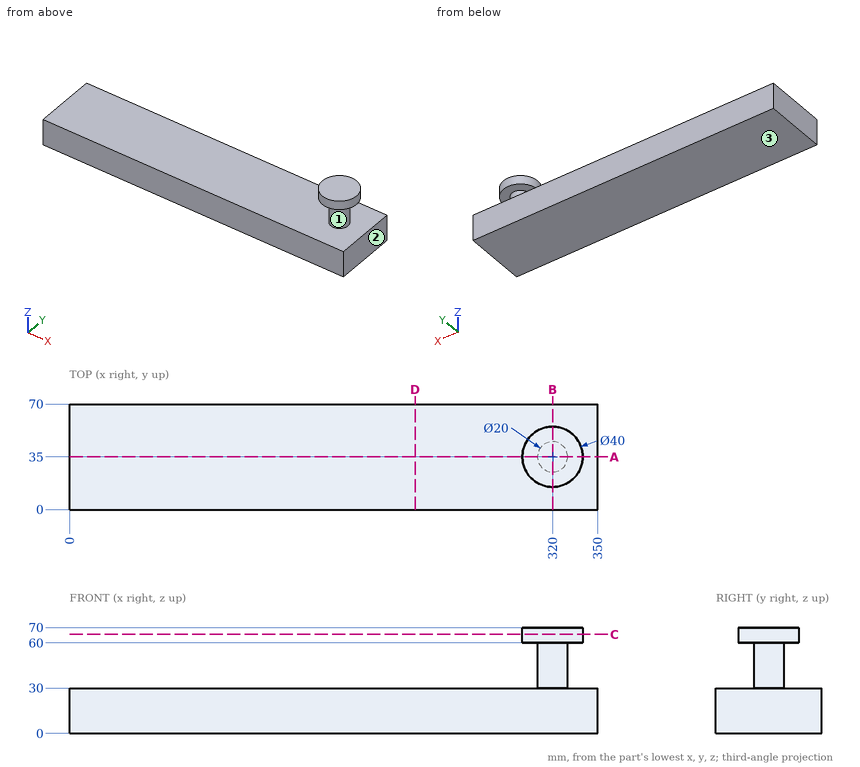
Here's the drawing with two shaded views (mm, measured from the low corner). I have some questions. Coordinates: 2 decimals unless noted, no trailing zeros. Order: outer loops, then holes, each group sorted by start corner. A loop starts at its lowest first (then second) coordinate and runs counter-clockwise, first axis right, second up. Notation, with made-up numbers: (-37, 69) - (19, 69) arc R19 cw to (19, 75) - close; hole circle Ø7 at (75, 61.5). An arc over 180 degrees is marked (long way). Answer in a Markdown table with one row per item. Add a question column.
(1) If we section it at D-D, the plane x = 229: Please give me the cut outline in (y, z), then the cut area to 3 significant figures.
(2) I need wall thicknesses on L1, parallel to Z at x = 318, y = 50; L2, parallel to Z at x = 100, y = 25.5; L3, parallel to X at y = 32.5, z = 32. Which ranges of each line are inside material? Lowest first, please.
(3) Will these pins go through, and if not, where does the flat tip stop? pin 1 (3 mm diameter, centred on x = 209.5, y = 46.5, fed in from +Z); pin 2 (1 mm diameter, centred on y = 32.5, z = 58.5, fed in from +X).
(4) If we section it at B-B, the plane x = 320: Please give me the cut outline in (y, z).
(5) If we mould it in two halves opening along Z, with no side actions, what happens to the marked faces 1, 2 and 3? For each: released by +Z, released by -Z, zero draft, split by the parting line, or undercut.
(6) If we section it at C-C, the plane z = 65.5: Please give me the cut outline in (x, y), then the cut area to 3 significant figures.
(7) If we section it at A-A, the plane y = 35: Please give me the cut outline in (x, z).
Results are:
| question | item | result |
|---|---|---|
| 1 | outline | (0, 0) - (70, 0) - (70, 30) - (0, 30) - close |
| 1 | area | 2,100 mm2 |
| 2 | L1 | z = 0 to 30, 60 to 70 |
| 2 | L2 | z = 0 to 30 |
| 2 | L3 | x = 310.32 to 329.68 |
| 3 | pin 1 | stops at z = 30 |
| 3 | pin 2 | stops at x = 329.8 |
| 4 | outline | (0, 0) - (70, 0) - (70, 30) - (45, 30) - (45, 60) - (55, 60) - (55, 70) - (15, 70) - (15, 60) - (25, 60) - (25, 30) - (0, 30) - close |
| 5 | face 1 | undercut |
| 5 | face 2 | zero draft |
| 5 | face 3 | released by -Z |
| 6 | outline | circle Ø40 at (320, 35) |
| 6 | area | 1,260 mm2 |
| 7 | outline | (0, 0) - (350, 0) - (350, 30) - (330, 30) - (330, 60) - (340, 60) - (340, 70) - (300, 70) - (300, 60) - (310, 60) - (310, 30) - (0, 30) - close |
